Build history of the part. All positions in model axes, mm. Face numbers are marked on the shaded views. Round coordinates to 2 decimals unless told otherwise and drop trailing zeros. Write each loop counter-clockwise with the first axis right and the second up, starting at its lowest first coordinate (ties: lowest second). Pieces come first, ordered by that corner, then holes. Notation, with made-up numbers: (63.5, -23.5) -> (113.5, -23.5) arc R9 cw to (113.5, -15.5) -> close; hole circle Ø3 at (10, 61.5). An arc over 180 degrees is marked (long way). Return JSON: item names as keys, results as strings.
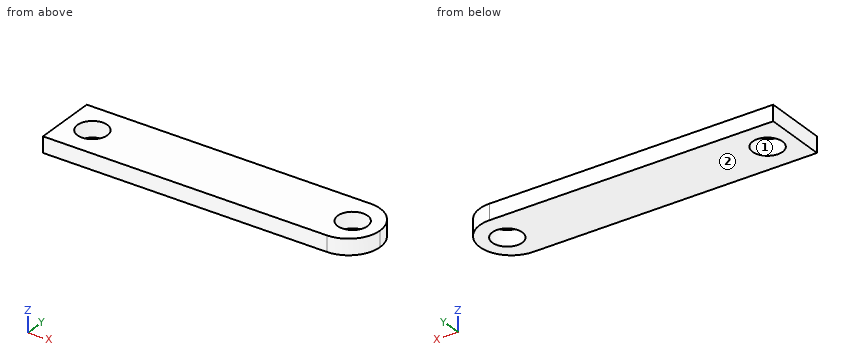
from build123d import *

# Parameters (mm, degrees)
F0_R     = 9.5
F1_DEPTH = 10


with BuildPart() as f1:
    # F0 (on Top) → F1 (new body)
    with BuildSketch(Plane.XY):
        with BuildLine():
            Line((-100, -20), (80, -20))
            ThreePointArc((80, -20), (94.142136, -14.142136), (100, 0))
            ThreePointArc((100, 0), (94.142136, 14.142136), (80, 20))
            Line((80, 20), (-100, 20))
            Line((-100, 20), (-100, -20))
        make_face()
        with Locations((-82.55, 0)):
            Circle(F0_R, mode=Mode.SUBTRACT)
        with Locations((82.55, 0)):
            Circle(F0_R, mode=Mode.SUBTRACT)
    extrude(amount=F1_DEPTH)


solid = f1.part
Q1. Wall check: L1, parallel to X at y = -4.5, z = 7.75; L2, parallel to Y at x = -82.55, z = 5; L3, parallel to X at y = -8, z = 5.75. Give the ranges that are in metal, low to high.
Verdict:
{"L1": "x = -100 to -90.92, -74.18 to 74.18, 90.92 to 99.49", "L2": "y = -20 to -9.5, 9.5 to 20", "L3": "x = -100 to -87.67, -77.43 to 77.43, 87.67 to 98.33"}
Q2. Saw through at B-B on x = -82.55. List the corners of the cut face in (y, z).
Verdict:
{"outline": "(-20, 0) -> (-9.5, 0) -> (-9.5, 10) -> (-20, 10) -> close; (9.5, 0) -> (20, 0) -> (20, 10) -> (9.5, 10) -> close"}
Q3. Two-plate mould, pull along X, no slides. Class the marked faces 1 and 2: +X half, -X half, draft (parallel to the pull), parting line (faces both ways), or undercut.
Verdict:
{"face 1": "undercut", "face 2": "draft"}
Q4. Saw through at A-A on z = 3. List the corners of the cut face in (x, y).
Verdict:
{"outline": "(-100, -20) -> (80, -20) arc R20 ccw to (100, 0) arc R20 ccw to (80, 20) -> (-100, 20) -> close; hole circle Ø19 at (-82.55, 0); hole circle Ø19 at (82.55, 0)"}
Q5. Saw through at D-D on y = -17. List the corners of the cut face in (x, z).
Verdict:
{"outline": "(-100, 0) -> (90.54, 0) -> (90.54, 10) -> (-100, 10) -> close"}
Q6. Pin check, flat tips, straight feed: pin 1 Ø10 at (x, y) = (-76.5, -15) entering from -Z; pin 2 Ø11.5 at (x, y) = (-82.55, 0) entering from +Z; pin 3 Ø5 at (y, z) = (7, 5) entering from +X. Stop position of each tip, or through.
Verdict:
{"pin 1": "stops at z = 0", "pin 2": "passes through", "pin 3": "stops at x = 99.49"}
Q7. Saw through at C-C on x = 82.55. List the corners of the cut face in (y, z).
Verdict:
{"outline": "(-19.84, 0) -> (-9.5, 0) -> (-9.5, 10) -> (-19.84, 10) -> close; (9.5, 0) -> (19.84, 0) -> (19.84, 10) -> (9.5, 10) -> close"}
